```python
from build123d import *

# Parameters (mm, degrees)
F1_DEPTH       = 15
F3_D           = 4.2
F3_DEPTH       = 10
F3_CSINK_D     = 6
F3_CSINK_ANGLE = 90
F3_TIP         = 1.2618073
F4_DEPTH       = 25


with BuildPart() as f1:
    # F0 (on Top) → F1 (new body)
    with BuildSketch(Plane.XY):
        with BuildLine():
            ThreePointArc((-48.4659095265, 39.8574409581), (-49.4215542208, 41.7790062675), (-49.9561374759, 43.8574409581))
            Line((-49.9561374759, 43.8574409581), (-52.9813081262, 43.8574409581))
            ThreePointArc((-52.9813081262, 43.8574409581), (-52.58380258, 41.8136904443), (-51.8710510318, 39.8574409581))
            Line((-51.8710510318, 39.8574409581), (-48.4659095265, 39.8574409581))
        make_face()
        with BuildLine():
            ThreePointArc((-51.8710510318, 39.8574409581), (-52.58380258, 41.8136904443), (-52.9813081262, 43.8574409581))
            Line((-52.9813081262, 43.8574409581), (-58.0664875805, 43.8574409581))
            Line((-58.0664875805, 43.8574409581), (-58.0664875805, 39.8574409581))
            Line((-58.0664875805, 39.8574409581), (-51.8710510318, 39.8574409581))
        make_face()
        with BuildLine():
            Line((-21.5664875805, 43.8574409581), (-26.6516670349, 43.8574409581))
            ThreePointArc((-26.6516670349, 43.8574409581), (-27.0491725811, 41.8136904443), (-27.7619241293, 39.8574409581))
            Line((-27.7619241293, 39.8574409581), (-21.5664875805, 39.8574409581))
            Line((-21.5664875805, 39.8574409581), (-21.5664875805, 43.8574409581))
        make_face()
        with BuildLine():
            ThreePointArc((-29.6768376852, 43.8574409581), (-37.682197339, 35.3321077883), (-48.4659095265, 39.8574409581))
            Line((-48.4659095265, 39.8574409581), (-51.8710510318, 39.8574409581))
            ThreePointArc((-51.8710510318, 39.8574409581), (-39.8164875805, 32.1074409581), (-27.7619241293, 39.8574409581))
            ThreePointArc((-27.7619241293, 39.8574409581), (-27.0491725811, 41.8136904443), (-26.6516670349, 43.8574409581))
            Line((-26.6516670349, 43.8574409581), (-29.6768376852, 43.8574409581))
        make_face()
    extrude(amount=F1_DEPTH)

    # F3
    with Locations(Plane.XZ.offset(-39.8574409581)):
        with Locations((-52.8164875805, 7.5), (-26.8164875805, 7.5)):
            CounterSinkHole(F3_D / 2, F3_CSINK_D / 2, depth=F3_DEPTH, counter_sink_angle=F3_CSINK_ANGLE)
            with Locations((0, 0, -(F3_DEPTH + F3_TIP / 2))):  # 118° drill point
                Cone(0, F3_D / 2, F3_TIP, mode=Mode.SUBTRACT)

    # F2 (on face) → F4 (cut)
    with BuildSketch(Plane.XZ.offset(-39.8574409581)):
        Polygon((-54.8949485496, 3.9), (-50.7380266115, 3.9), (-48.6595656424, 7.5), (-50.7380266115, 11.1), (-54.8949485496, 11.1), (-56.9734095187, 7.5), align=None)
        Polygon((-28.8949485496, 3.9), (-24.7380266115, 3.9), (-22.6595656424, 7.5), (-24.7380266115, 11.1), (-28.8949485496, 11.1), (-30.9734095187, 7.5), align=None)
    extrude(amount=F4_DEPTH, mode=Mode.SUBTRACT)


solid = f1.part
```
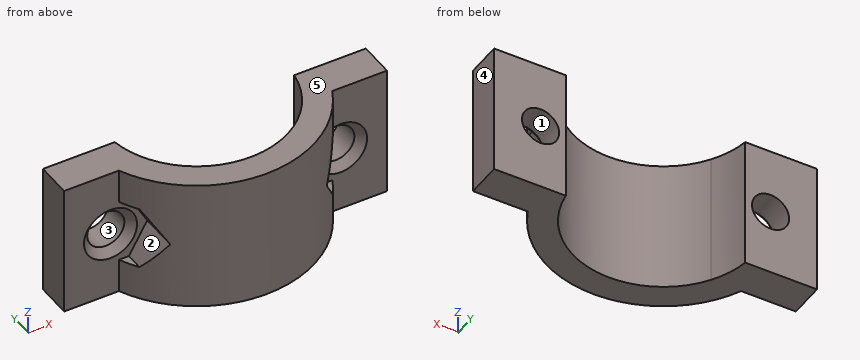
Here's how the part is built. I have some questions about the finished solid (model axes, mm). Face numbers are marked on the shaded views. A direction names the side the tool comes from. Give positions to 0.01 mm unless a question says otherwise; leave off trailing zeros. Order: outer loops, then holes, each group sorted by start corner. A loop starts at its lowest first (then second) coordinate and runs counter-clockwise, first axis right, second up. Notation, with made-up numbers: M 89,77 L 111,77 A37 cw 111,116 Z; hole C 88,-8 d7. An arc over 180 degrees is marked long. Use a Markdown table: item, result. Add a question column.
1. Suppose I cut it at D-D (z = 8). Give the number of separate pieces and of enclosed holes in the cut face, and give its area (3 significant figures).
2. For pin 1 Ø7.5 at (x, z) = (-27.5, 11) entering from -Y; pin 2 Ø2.5 at (x, z) = (-52.82, 7.5) entering from -Y; pin 3 Ø5 at (x, z) = (-46, 4.5) entering from -Y; pin 4 Ø3 at (x, z) = (-43.5, 10) entering from +Y, each with a flat end and sliding along its axis, tell me the tip position at first contact or that it passes through.
3. Suppose I cut it at A-A (y = 41.75). List the corners of the cut face in (x, z) for me, and give its area (3 significant figures).
4. I need wall thicknesses on probe 1 along Z at (x, y) = (-27, 42); probe 2 along X at (y, z) = (43, 7.5); probe 3 along X at (y, z) = (42.55, 7.5). Which ranges of each line are inside material? Lowest first, please. Write a range as from..to.
5. Suppose I cut it at C-C (y = 38.25). List the corners of the cut face in (x, z) for me, and give its area (3 significant figures).
6. Suppose I cut it at B-B (z = 2). List the corners of the cut face in (x, y) for me, and give its area (3 significant figures).
7. If we mould it in two halves opening along Z, with no side actions, what happens to the marked faces 3, 4 and 5? For each: +Z half, -Z half, draft (parallel to the pull), parting line (faces both ways), or undercut.
8. On a 3-axis mill with a long thin cutter (end or side, diameter ignored), from which of +Z, -Z, +X, -X, +Y, -Y can I reach the whole of each face in a straight line? I mean the marked faces 1 and 2. Say none if no direction works.
Results list:
| question | item | result |
|---|---|---|
| 1 | separate pieces | 3 |
| 1 | enclosed holes | 0 |
| 1 | area | 98.0 mm² |
| 2 | pin 1 | stops at y = 35.25 |
| 2 | pin 2 | passes through |
| 2 | pin 3 | stops at y = 32.63 |
| 2 | pin 4 | stops at y = 36.51 |
| 3 | outline | M -58.07,0 L -49.41,0 L -49.41,15 L -58.07,15 Z; M -30.22,0 L -21.57,0 L -21.57,15 L -30.22,15 Z; hole C -52.82,7.5 d4.2; hole C -26.82,7.5 d4.2 |
| 3 | area | 232 mm² |
| 4 | probe 1 | z = 0..5.41, 9.59..15 |
| 4 | probe 2 | x = -58.07..-54.92, -50.72..-49.79, -29.84..-28.92, -24.72..-21.57 |
| 4 | probe 3 | x = -58.07..-54.92, -50.72..-49.67, -29.96..-28.92, -24.72..-21.57 |
| 5 | outline | M -51,0 L -47.2,0 L -47.2,15 L -51,15 L -51,11.1 L -50.74,11.1 L -48.66,7.5 L -50.74,3.9 L -51,3.9 Z; M -32.43,0 L -28.63,0 L -28.63,3.9 L -28.89,3.9 L -30.97,7.5 L -28.89,11.1 L -28.63,11.1 L -28.63,15 L -32.43,15 Z |
| 5 | area | 95.2 mm² |
| 6 | outline | M -58.07,39.86 L -51.87,39.86 A13.25 ccw -27.76,39.86 L -21.57,39.86 L -21.57,43.86 L -29.68,43.86 A10.25 cw -49.96,43.86 L -58.07,43.86 Z |
| 6 | area | 146 mm² |
| 7 | face 3 | undercut |
| 7 | face 4 | draft |
| 7 | face 5 | +Z half |
| 8 | face 1 | +Y, -Y |
| 8 | face 2 | -X, -Y |
